```python
from build123d import *

# Parameters (mm, degrees)
SKETCH_2_W           = 26
SKETCH_2_H           = 97
EXTRUDE_1_DEPTH      = 10
CUT_EXTRUDE_11_DEPTH = 10
EXTRUDE_2_DEPTH      = 3
SKETCH_8_R           = 2
CUT_EXTRUDE_12_DEPTH = 3
EXTRUDE_3_DEPTH      = 5
CUT_EXTRUDE_START    = -10
SKETCH_10_R          = 2
CUT_EXTRUDE_13_DEPTH = 10
EXTRUDE_4_DEPTH      = 10
EXTRUDE_5_DEPTH      = 10
EXTRUDE_6_DEPTH      = 8


with BuildPart() as part:
    # 草图2 → 凸台-拉伸1 (new body)
    with BuildSketch(Plane.XY):
        with Locations((0, -10.25)):
            Rectangle(SKETCH_2_W, SKETCH_2_H)
    extrude(amount=EXTRUDE_1_DEPTH)

    # 草图3 → 切除-拉伸11 (cut)
    with BuildSketch(Plane.XY):
        with BuildLine():
            Line((-11, -2.75), (-11, 25.25))
            ThreePointArc((-11, 25.25), (0, 36.25), (11, 25.25))
            Line((11, 25.25), (11, -2.75))
            ThreePointArc((11, -2.75), (0, -13.75), (-11, -2.75))
        make_face()
    extrude(amount=CUT_EXTRUDE_11_DEPTH, mode=Mode.SUBTRACT)

    # 草图4 → 凸台-拉伸2 (add)
    with BuildSketch(Plane.XZ.offset(58.75)):
        Polygon((-13, 0), (37, 0), (37, 16), (-3, 54), (-13, 54), align=None)
    extrude(amount=EXTRUDE_2_DEPTH)

    # 草图8 → 切除-拉伸12 (cut)
    with BuildSketch(Plane.XZ.offset(61.75)):
        with Locations(Location((-5.5, 49.5, 0), (0, 0, 270))):
            Circle(SKETCH_8_R)
    extrude(amount=-CUT_EXTRUDE_12_DEPTH, mode=Mode.SUBTRACT)

    # 草图9 → 凸台-拉伸3 (add)
    with BuildSketch(Plane(origin=(0, -58.75, 0), x_dir=(1, 0, 0), z_dir=(0, 1, 0))):
        Polygon((-13, -10), (-13, -54), (-3, -54), (37, -16), (37, 0), (13, 0), (13, -10), align=None)
    extrude(amount=EXTRUDE_3_DEPTH)

    # 草图10 → 切除-拉伸13 (cut)
    with BuildSketch(Plane(origin=(0, -53.75, 0), x_dir=(1, 0, 0), z_dir=(0, 1, 0)).offset(CUT_EXTRUDE_START)):
        with Locations(Location((-5.5, -49.5, 0), (0, 0, 90))):
            Circle(SKETCH_10_R)
    extrude(amount=CUT_EXTRUDE_13_DEPTH, mode=Mode.SUBTRACT)

    # 草图11 → 凸台-拉伸4 (add)
    with BuildSketch(Plane(origin=(0, 0, 0), x_dir=(-1, 0, 0), z_dir=(0, 0, -1))):
        Polygon((-13, -33.75), (-13, -53.75), (-25, -53.75), align=None)
    extrude(amount=-EXTRUDE_4_DEPTH)

    # 草图12 → 凸台-拉伸5 (add)
    with BuildSketch(Plane.ZY.offset(13)):
        Polygon((10, -53.75), (35, -53.75), (10, -33.75), align=None)
    extrude(amount=-EXTRUDE_5_DEPTH)

    # 草图13 → 凸台-拉伸6 (add)
    with BuildSketch(Plane(origin=(0, -53.75, 0), x_dir=(1, 0, 0), z_dir=(0, 1, 0))):
        Polygon((37, 0), (42, 0), (42, -11), (37, -16), align=None)
    extrude(amount=-EXTRUDE_6_DEPTH)


solid = part.part
```
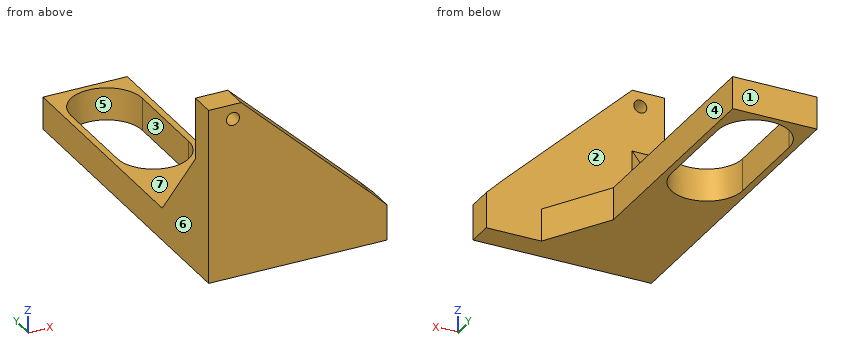
Part model, mm, in its own coordinate system. Face numbers are marked on the shaded views. A direction names the side the tool comes from. Coordinates: 2 decimals unless noted, no trailing zeros. Order: outer loops, then holes, each group sorted by start corner. A loop starts at its lowest first (then second) coordinate and runs counter-clockwise, first axis right, second up. Notation, with made-up numbers: (65.25, -13.5) -> (99.25, -13.5) arc R12 cw to (99.25, 8.5) -> close; hole circle Ø4 at (57, 74.5). An arc over 180 degrees is marked (long way). Put each result on its own line as item: value. Start each with the question number.
(1) Band-saw the part on D-D (x = -5.5). Give the cut face in (y, z), then the cut area to 3 significant figures.
(2) Probe line 1 along Z through (x, y) = (-5.5, -59.5); line 2 along X through (y, z) = (23.5, 7.5); line 3 along Y through (x, z) = (5.5, 36). List the from-to ranges inside material, lowest first. Write a range as [from, to].
(3) Which spindle directions (+Z, -Z, +X, -X, +Y, -Y) get a long thin tool onto all of the face, cutting with end or side? Do the marked faces 1, 2, 3 and 4. Say none if no direction does.
(4) Pin check, flat tips, straight feed: pin 1 Ø1 at (x, z) = (29, 24) entering from -Y; pin 2 Ø8 at (x, y) = (30.5, -49) entering from -Z; pin 3 Ø11 at (y, z) = (17, 2.5) entering from +X; pin 4 Ø5 at (x, z) = (-3, 40.5) entering from +Y. Stop position of each tip, or through.
(5) Mould opens along X. For the marked faces 5, 6 and 7 say: pulls with the +X half, pulls with the -X half, needs draft (parallel to the pull), parting line crosses it, or undercut.
(6) Band-saw the part on C-C (z = 49.5). Give the cut face in (x, y).
(7) Band-saw the part on A-A (y = 4.5). Give the cut face in (x, z).
(8) Band-saw the part on B-B (x = 0). Give the cut face in (y, z), then the cut area to 3 significant figures.
Determined:
1. outline: (-61.75, 0) -> (-12.28, 0) -> (-12.28, 10) -> (-33.75, 10) -> (-53.75, 35) -> (-53.75, 47.5) -> (-61.75, 47.5) -> close; (-61.75, 51.5) -> (-53.75, 51.5) -> (-53.75, 54) -> (-61.75, 54) -> close; (34.78, 0) -> (38.25, 0) -> (38.25, 10) -> (34.78, 10) -> close
1. area: 1,100 mm²
2. line 1: z = [0, 47.5], [51.5, 54]
2. line 2: x = [-13, -11], [11, 13]
2. line 3: y = [-61.75, -53.75]
3. face 1: +Z, -Z, +X, -X, +Y
3. face 2: +Z, +X, +Y
3. face 3: +Z, -Z
3. face 4: +Z, -Z, +X, +Y
4. pin 1: stops at y = -61.75
4. pin 2: passes through
4. pin 3: stops at x = 13
4. pin 4: stops at y = -53.75
5. face 5: undercut
5. face 6: pulls with the -X half
5. face 7: needs draft
6. outline: (-13, -61.75) -> (-7.5, -61.75) -> (-7.5, -53.75) -> (-13, -53.75) -> close; (-3.5, -61.75) -> (1.74, -61.75) -> (1.74, -53.75) -> (-3.5, -53.75) -> close
7. outline: (-13, 0) -> (-11, 0) -> (-11, 10) -> (-13, 10) -> close; (11, 0) -> (13, 0) -> (13, 10) -> (11, 10) -> close
8. outline: (-61.75, 0) -> (-13.75, 0) -> (-13.75, 10) -> (-53.75, 10) -> (-53.75, 51.15) -> (-61.75, 51.15) -> close; (36.25, 0) -> (38.25, 0) -> (38.25, 10) -> (36.25, 10) -> close
8. area: 829 mm²
